Source: three-view drawing plus pictorial views. Frame: mm from the lowest corner of the part. A direction names the side the tool comes from. Round coordinates to 2 decimals unless told otherwise and drop trailing zeros. Loops run counter-clockwise (first coordinate to the right, second up) from the corner with the lowest first, then second, coordinate; pieces in that order, holes last. Notation, with made-up numbers: M 22,3 L 65,3 A34 ccw 65,38 Z; hole C 29.25,44.25 d9. An arc over 180 degrees is marked long. Answer as a JSON object with one key per item and string values.
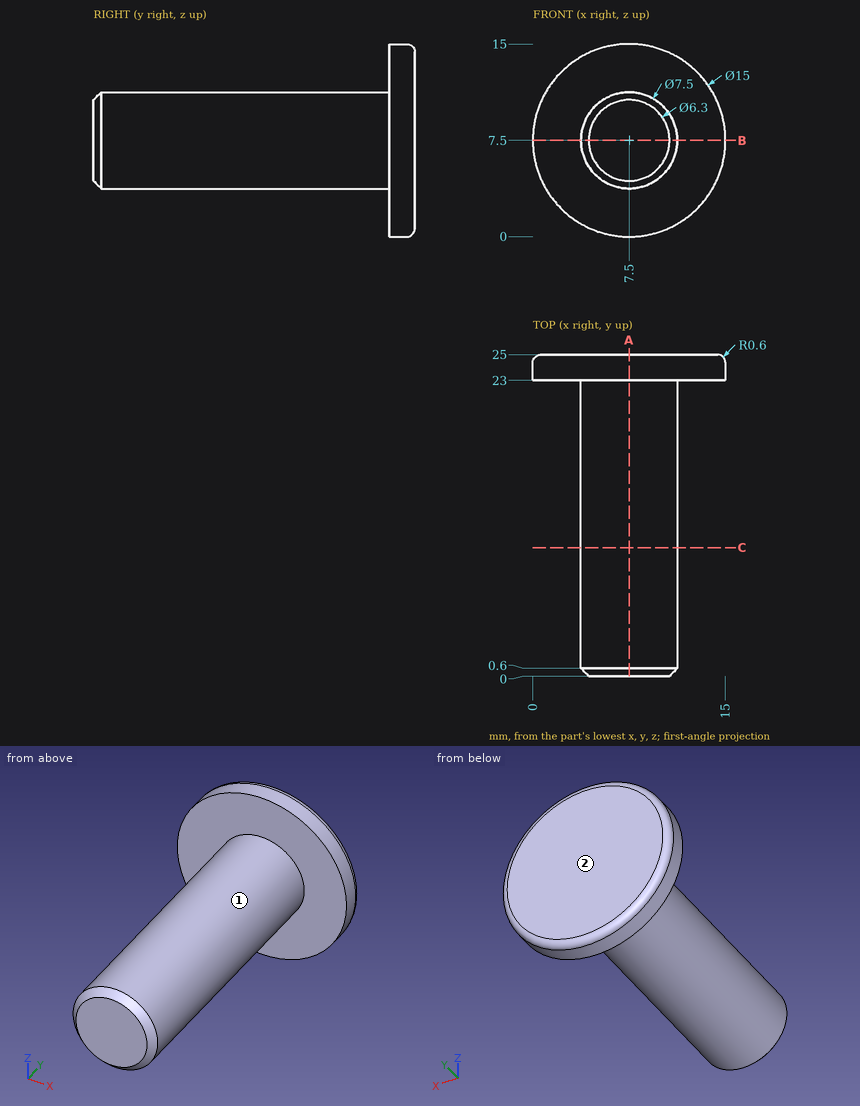
1) First-contact query: pin 1 (6 mm diameter, centred on x = 7, y = 13.5, fed in from +Z); pin 2 (8 mm diameter, centred on x = 11.5, z = 9.5, fed in from -Y); pin 3 (8 mm diameter, centred on y = 20, z = 4, fed in from -X); pin 4 (3 mm diameter, centred on x = 12, y = 13, fed in from -Z). Flat tips, straight axial feed; report the tip coordinate or a pass-through.
Geometry results:
{"pin 1": "z = 11.25", "pin 2": "y = 0", "pin 3": "x = 0.05", "pin 4": "z = 5.25"}
2) Line query: probe 1 along Y at (x, z) = (4.75, 12.75); probe 2 along Z at (x, y) = (4.25, 22.5); probe 3 along Z at (x, y) = (10.25, 23.5). Output: solid intervals per line, ascending.
Geometry results:
{"probe 1": "23 to 25", "probe 2": "5.63 to 9.37", "probe 3": "0.52 to 14.48"}
3) Cut plane B-B on z = 7.5. Return the cut outline in (x, y).
Geometry results:
{"outline": "M 0,23 L 3.75,23 L 3.75,0.6 L 4.35,0 L 10.65,0 L 11.25,0.6 L 11.25,23 L 15,23 L 15,24.4 A0.6 ccw 14.4,25 L 0.6,25 A0.6 ccw 0,24.4 Z"}
4) Cut plane C-C on y = 10. Return the cut outline in (x, z), and give its area (3 significant figures).
Geometry results:
{"outline": "C 7.5,7.5 d7.5", "area": "44.2 mm2"}
5) Set-up query: the marked faces 1 and 2. Return all of +Z, -Z, +X, -X, +Y, -Y with unobstructed straight access to the full face (end or side cutting, diameter ignored); none if empty.
Geometry results:
{"face 1": "-Y", "face 2": "+Z, -Z, +X, -X, +Y"}
6) Cut plane A-A on x = 7.5. Return the cut outline in (y, z).
Geometry results:
{"outline": "M 0,4.35 L 0.6,3.75 L 23,3.75 L 23,0 L 24.4,0 A0.6 ccw 25,0.6 L 25,14.4 A0.6 ccw 24.4,15 L 23,15 L 23,11.25 L 0.6,11.25 L 0,10.65 Z"}
